Work out the finished part from the listing and answer in its coordinate system (mm). Face numbers are marked on the shaded views. A direction names the side the tool comes from. Round coordinates to 2 decimals unless told otherwise and drop trailing zeros. Order: outer loops, then holes, each group sorted by start corner. A loop starts at its lowest first (then second) coordinate and runs counter-clockwise, first axis right, second up. Notation, with made-up numbers: (18, 21.5) - (28, 21.5) arc R25 ccw to (28, 39.5) - close; hole circle Ø7 at (35, 33.5). An arc over 180 degrees is marked (long way). Put each result on its own line as item: value.
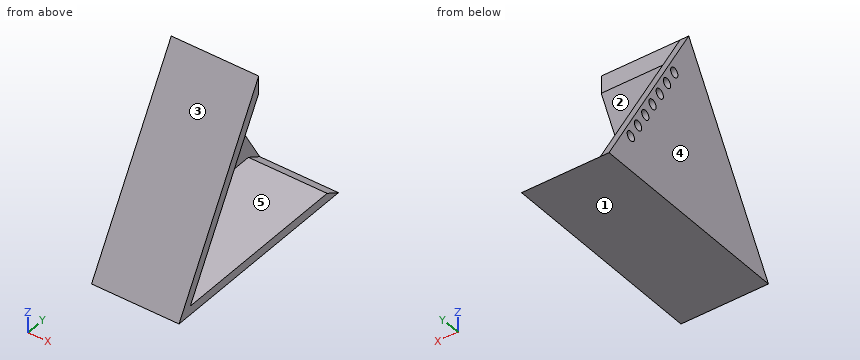
```python
from build123d import *

# Parameters (mm, degrees)
F1_DEPTH = 45
F2_T     = -4.5
F4_D     = 5
F4_DEPTH = 12
F4_TIP   = 1.5021515476
F6_DEPTH = 40.5


with BuildPart() as f1:
    # F0 (on Right) → F1 (new body)
    with BuildSketch(Plane.YZ):
        Polygon((-46.7345683003, 84.126270037), (-101.7345683003, -11.1365243793), (8.2654316997, -11.1365243793), align=None)
    extrude(amount=F1_DEPTH)

    # F2
    f2_openings = [f1.faces().sort_by_distance(p)[0] for p in [
        (45, -46.734568, 20.61774),
    ]]
    offset(amount=F2_T, openings=f2_openings)

    # F4
    with Locations(Plane(origin=(0, 0, 0), x_dir=(0, -1, 0), z_dir=(-1, 0, 0))):
        with Locations((36.7409650803, 58.8168415093), (31.7409650803, 50.1565874715), (26.7409650803, 41.4963334336), (21.7409650803, 32.8360793958), (16.7409650803, 24.1758253579), (11.7409650803, 15.5155713201), (6.7409650803, 6.8553172823)):
            Hole(F4_D / 2, depth=F4_DEPTH)
            with Locations((0, 0, -(F4_DEPTH + F4_TIP / 2))):  # 118° drill point
                Cone(0, F4_D / 2, F4_TIP, mode=Mode.SUBTRACT)

    # F5 (on face) → F6 (cut, symmetric)
    with BuildSketch(Plane.YZ.offset(45)):
        Polygon((-46.7345683003, 84.126270037), (-46.7345683003, 75.126270037), (0.4712030657, -6.6365243793), (8.2654316997, -11.1365243793), align=None)
    extrude(amount=F6_DEPTH, both=True, mode=Mode.SUBTRACT)


solid = f1.part
```
1) A cutting plane is placed at B-B on y = -71. Write down the section's boundary in (x, z), then the cut area to 3 significant figures.
Findings below:
outline: (0, -11.14) - (45, -11.14) - (45, -6.64) - (4.5, -6.64) - (4.5, 33.1) - (45, 33.1) - (45, 42.1) - (0, 42.1) - close
area: 786 mm2
2) Straight lines are drawn through the part: L1, parallel to X at y = -69.5, z = 21; L2, parallel to Z at x = 34, y = -73; L3, parallel to Z at x = 5, y = -4. For each, find the intervals that lie inside material, in ascending order. Write a range as from..to.
Findings below:
L1: x = 0..4.5
L2: z = -11.14..-6.64, 29.63..38.63
L3: z = -11.14..-6.64
3) Given pin 1 Ø1.5 at (x, z) = (5, 9) entering from -Y; pin 2 Ø12 at (x, z) = (21, 70) entering from +Y; pin 3 Ø6 at (x, y) = (21, -6.5) entering from +Z; pin 4 Ø4.5 at (y, z) = (-16.74, 24.18) entering from +X, each flat-ended and moving along its own axis, determine where each tip first touches the part or whether it passes through.
Findings below:
pin 1: stops at y = -90.54
pin 2: stops at y = -46.73
pin 3: stops at z = -6.64
pin 4: passes through
4) For the marked faces 1 and 2, determine the directions among +Z, -Z, +X, -X, +Y, -Y from which every point of the face is accessible in a straight line to the end or side of a thin tool.
Findings below:
face 1: -Z, +X, -X, +Y, -Y
face 2: +X, +Y
5) A cutting plane is placed at C-C on z = 78. Write down the section's boundary in (x, y).
Findings below:
outline: (0, -50.27) - (45, -50.27) - (45, -46.73) - (4.5, -46.73) - (4.5, -43.2) - (0, -43.2) - close
6) For a pull along Z with two mould halves and no side action, classify the marked faces 3, 4 and 5 as pulls with the +Z half, pulls with the -Z half, needs draft (parallel to the pull), parting line crosses it, or undercut.
Findings below:
face 3: pulls with the +Z half
face 4: needs draft
face 5: undercut
7) A cutting plane is placed at A-A on x = 23. Write down the section's boundary in (y, z).
Findings below:
outline: (-101.73, -11.14) - (8.27, -11.14) - (0.47, -6.64) - (-93.94, -6.64) - (-46.73, 75.13) - (-46.73, 84.13) - close
